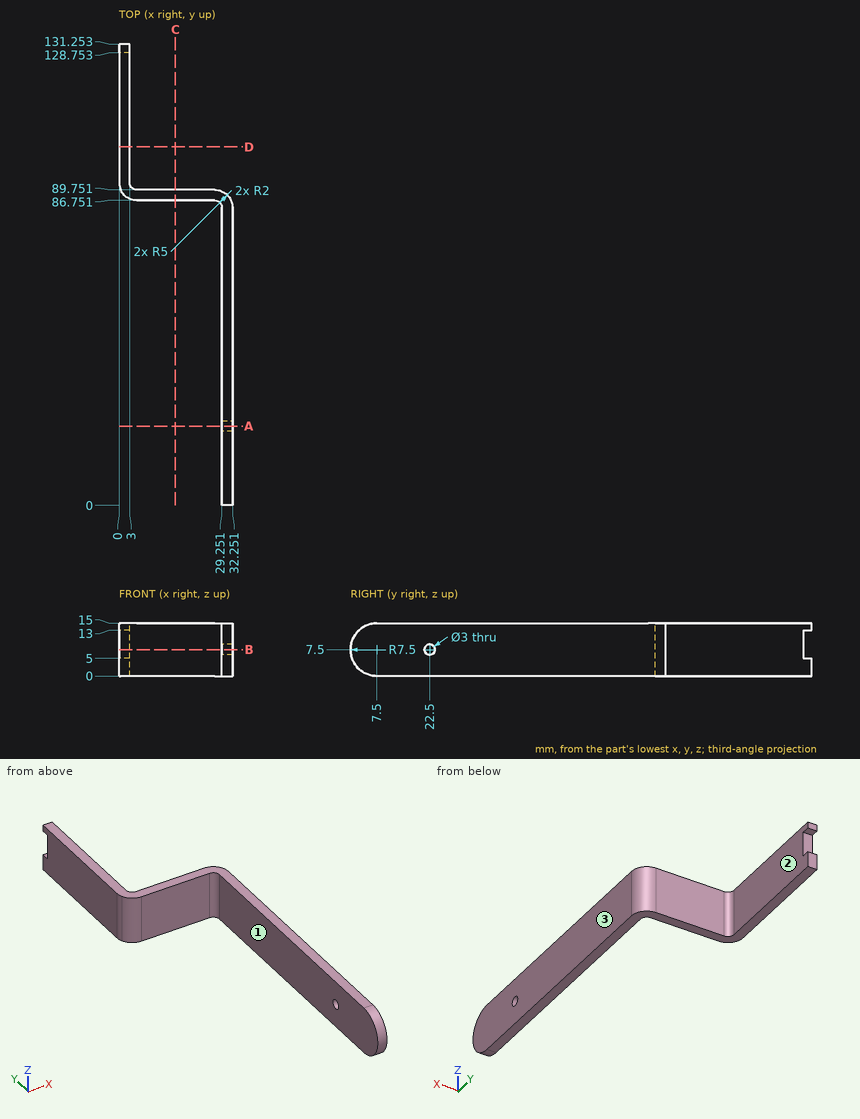
Print and shaded views of the part. All mm, measured from the part's lowest x, y and z. A direction names the side the tool comes from. Round coordinates to 2 decimals unless told otherwise and drop trailing zeros. Write each loop counter-clockwise with the first axis right and the second up, starting at its lowest first coordinate (ties: lowest second). Pieces come first, ordered by that corner, then holes. Notation, with made-up numbers: (60, 37) -> (105, 37) arc R15 ccw to (105, 43) -> close; hole circle Ø9 at (-33.5, 48.25). An arc over 180 degrees is marked (long way). Return JSON: item names as keys, results as strings. Group by question number.
Q1. Saw through at D-D on y = 102. Write the cut outline in (x, z).
Q2. Saw through at B-B on z = 7.5. Write the cut outline in (x, y), plus the area to 3 significant figures.
Q3. Pin check, flat tips, straight feed: pin 1 (8 mm diameter, centred on x = 6.5, z = 7.5, fed in from -Y); pin 2 (4 mm diameter, centred on y = 25, z = 13, fed in from -X); pin 3 (2.5 mm diameter, centred on y = 22.5, z = 7.5, fed in from -X); pin 4 (0.9 mm diameter, centred on x = 1, z = 10.5, fed in from +Y). Stop position of each tip, or through.
Q4. Which spindle directions (+Z, -Z, +X, -X, +Y, -Y) get a long thin tool onto all of the face, cutting with end or side? Do the marked faces 1, 2 and 3. Say none if no direction does.
Q5. Saw through at A-A on y = 22.5. Write the cut outline in (x, z), plus the area to 3 significant figures.
Q6. Saw through at C-C on x = 16. Write the cut outline in (y, z).
Q7. Probe L1, parallel to Z at x = 30.25, y = 22.5; L2, parallel to Y at x = 22, z = 1.25; L3, parallel to X at y = 98.5, z = 6.75. List the from-to ranges inside material, lowest first. Write a range as [from, to].
Answer:
{
 "1": {"outline": "(0, 0) -> (3, 0) -> (3, 15) -> (0, 15) -> close"},
 "2": {"outline": "(0, 91.75) arc R5 ccw to (5, 86.75) -> (27.25, 86.75) arc R2 cw to (29.25, 84.75) -> (29.25, 24) -> (32.25, 24) -> (32.25, 84.75) arc R5 ccw to (27.25, 89.75) -> (5, 89.75) arc R2 cw to (3, 91.75) -> (3, 128.75) -> (0, 128.75) -> close; (29.25, 0) -> (32.25, 0) -> (32.25, 21) -> (29.25, 21) -> close", "area": "456 mm2"},
 "3": {"pin 1": "y = 86.75", "pin 2": "x = 29.25", "pin 3": "through", "pin 4": "y = 128.75"},
 "4": {"face 1": "+Z, -Z, -X, -Y", "face 2": "+Z, -Z, +X, +Y", "face 3": "+Z, -Z, +X, +Y, -Y"},
 "5": {"outline": "(29.25, 0) -> (32.25, 0) -> (32.25, 6) -> (29.25, 6) -> close; (29.25, 9) -> (32.25, 9) -> (32.25, 15) -> (29.25, 15) -> close", "area": "36.0 mm2"},
 "6": {"outline": "(86.75, 0) -> (89.75, 0) -> (89.75, 15) -> (86.75, 15) -> close"},
 "7": {"L1": "[0, 6], [9, 15]", "L2": "[86.75, 89.75]", "L3": "[0, 3]"}
}
